Can you work these out from the drawing? Everything is in mm from the part's minimum corner. A direction names the side the tool comes from. Round coordinates to 2 decimals unless told otherwise and drop trailing zeros. Loops run counter-clockwise (first coordinate to the right, second up) from the corner with the lowest first, then second, coordinate; pieces in that order, holes last. Notation, with made-up numbers: M 5.25,-10.75 L 36.25,-10.75 A16 cw 36.25,-6.75 Z; hole C 48,57 d6. An arc over 180 degrees is marked long. Use a Markdown table: item, result.
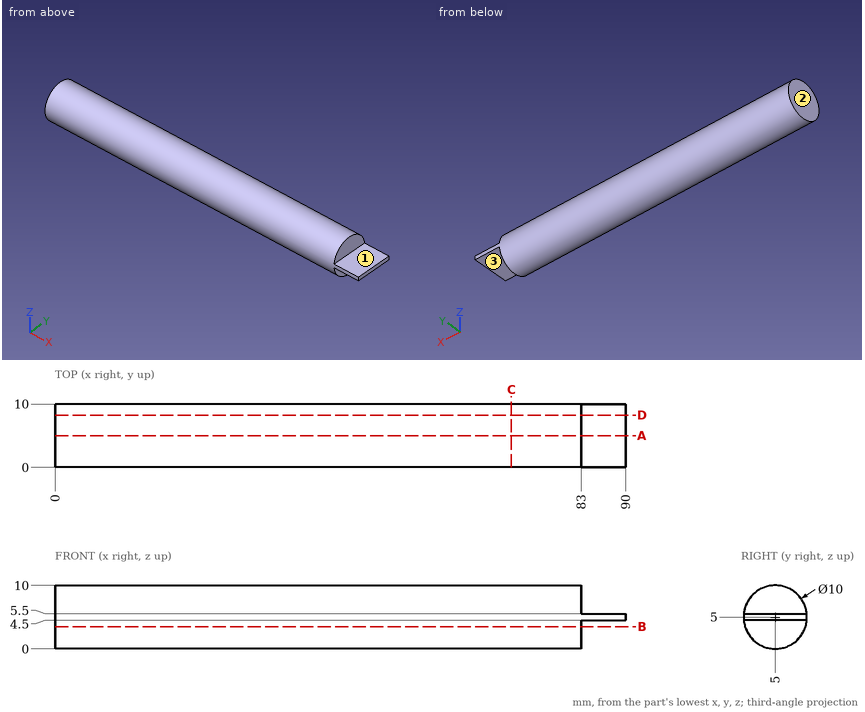
Q1. Imagine slicing it at D-D, the plane y = 8.25. Please give me the cut outline in (x, z).
Return value:
| item | result |
|---|---|
| outline | M 0,1.2 L 83,1.2 L 83,4.5 L 90,4.5 L 90,5.5 L 83,5.5 L 83,8.8 L 0,8.8 Z |
Q2. I need wall thicknesses on line 1 (X direction, y = 3.25, z = 9); line 2 (Y direction, x = 76, z = 4.75); line 3 (Z direction, x = 40.5, y = 6.5). Which ranges of each line are inside material? Lowest first, please. Write a range as from..to.
Return value:
| item | result |
|---|---|
| line 1 | x = 0..83 |
| line 2 | y = 0.01..9.99 |
| line 3 | z = 0.23..9.77 |
Q3. Imagine slicing it at B-B, the plane z = 3.5. Please give me the cut outline in (x, y).
Return value:
| item | result |
|---|---|
| outline | M 0,0.23 L 83,0.23 L 83,9.77 L 0,9.77 Z |
Q4. Will these pins go through, and if not, where does the flat tip stop? P1, Ø3.5, axis at y = 6.5, z = 2, coming from the +X side; P2, Ø1.5, axis at x = 37, y = 5.5, coming from the +Z side; P3, Ø6, axis at x = 30.5, z = 1.5, coming from the +Y side; P4, Ø2, axis at x = 85, y = 5, coming from the +Z side.
Return value:
| item | result |
|---|---|
| P1 | stops at x = 83 |
| P2 | stops at z = 10 |
| P3 | stops at y = 9.97 |
| P4 | stops at z = 5.5 |
Q5. Imagine slicing it at A-A, the plane y = 5. Please give me the cut outline in (x, z).
Return value:
| item | result |
|---|---|
| outline | M 0,0 L 83,0 L 83,4.5 L 90,4.5 L 90,5.5 L 83,5.5 L 83,10 L 0,10 Z |
Q6. Imagine slicing it at C-C, the plane x = 72. Please give me the cut outline in (y, z), then the cut area to 3 significant figures.
Return value:
| item | result |
|---|---|
| outline | C 5,5 d10 |
| area | 78.5 mm^2 |
Q7. For the marked faces 1, 2 and 3, which set-ups out of +Z, -Z, +X, -X, +Y, -Y let a thin tool reach every point of the face, with its end or its side?
Return value:
| item | result |
|---|---|
| face 1 | +Z, +X, +Y, -Y |
| face 2 | +Z, -Z, -X, +Y, -Y |
| face 3 | -Z, +X, +Y, -Y |
